Study the drawing (mm; zero at the part's minimum x, y, z) and answer. A direction names the side the tool comes from. Coordinates: 2 decimals unless noted, no trailing zeros. Order: outer loops, then holes, each group sorted by start corner. A loop starts at its lowest first (then second) coordinate and runs counter-clockwise, first axis right, second up. Notation, with made-up numbers: (53.5, 38) -> (59.5, 38) arc R27 cw to (59.5, 69) -> close; hole circle Ø11 at (53.5, 31). An arc over 180 degrees is marked (long way). One line per question, with ' | ' between items.
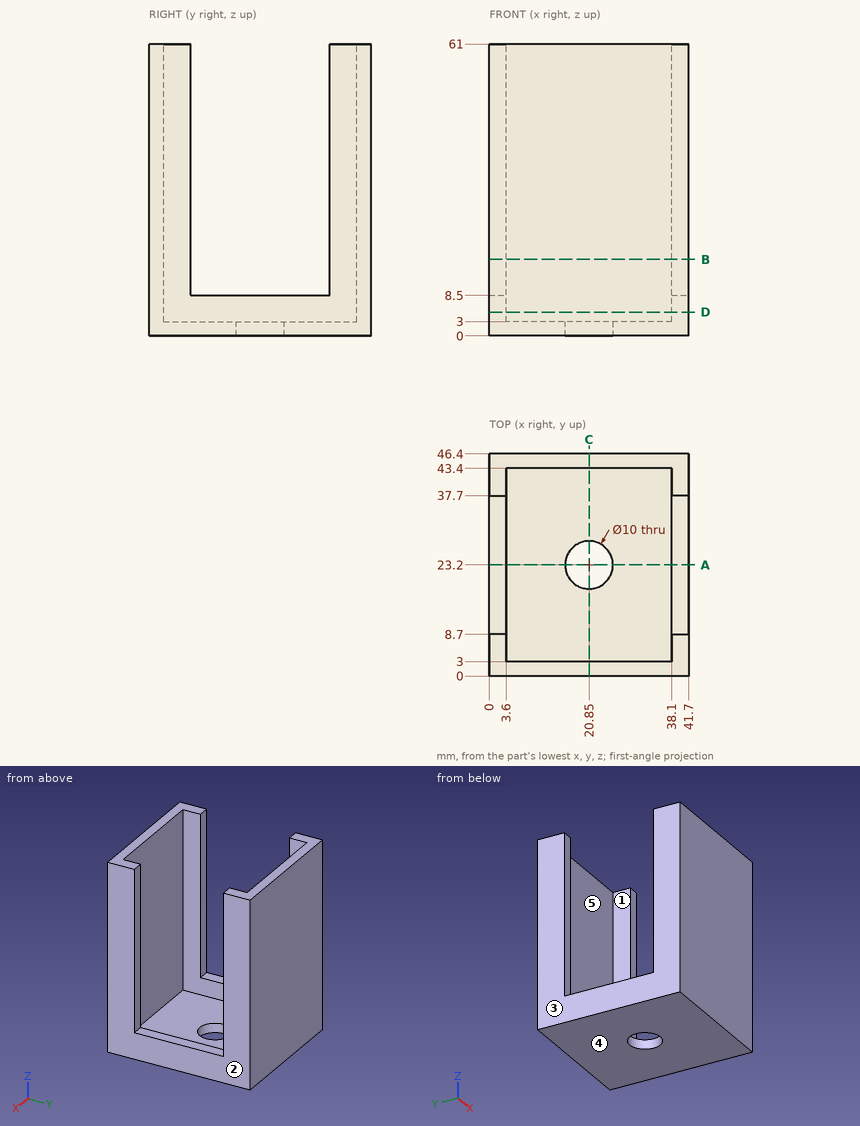
Item 1: Section A-A, the plane y = 23.2 is taken. Give the vertices of the cut face in (x, z), plus the area to 3 significant figures.
Computed values:
outline: (0, 0) -> (15.85, 0) -> (15.85, 3) -> (3.6, 3) -> (3.6, 8.5) -> (0, 8.5) -> close; (25.85, 0) -> (41.7, 0) -> (41.7, 8.5) -> (38.1, 8.5) -> (38.1, 3) -> (25.85, 3) -> close | area: 135 mm^2
Item 2: Section B-B, the plane z = 16 is taken. Give the vertices of the cut face in (x, y).
Computed values:
outline: (0, 0) -> (41.7, 0) -> (41.7, 8.7) -> (38.1, 8.7) -> (38.1, 3) -> (3.6, 3) -> (3.6, 8.7) -> (0, 8.7) -> close; (0, 37.7) -> (3.6, 37.7) -> (3.6, 43.4) -> (38.1, 43.4) -> (38.1, 37.7) -> (41.7, 37.7) -> (41.7, 46.4) -> (0, 46.4) -> close
Item 3: Each of these flat-tipped pins is pushed along its axis until it touches: pin 1 Ø3 at (x, y) = (2, 26.5) entering from +Z; pin 2 Ø8 at (x, y) = (27, 27) entering from +Z. Where does it stop, or does it pass through?
Computed values:
pin 1: stops at z = 8.5 | pin 2: stops at z = 3
Item 4: Section C-C, the plane x = 20.85 is taken. Give the vertices of the cut face in (y, z), plus the area to 3 significant figures.
Computed values:
outline: (0, 0) -> (18.2, 0) -> (18.2, 3) -> (3, 3) -> (3, 61) -> (0, 61) -> close; (28.2, 0) -> (46.4, 0) -> (46.4, 61) -> (43.4, 61) -> (43.4, 3) -> (28.2, 3) -> close | area: 457 mm^2
Item 5: Section D-D, the plane z = 5 is taken. Give the vertices of the cut face in (x, y), plus the area to 3 significant figures.
Computed values:
outline: (0, 0) -> (41.7, 0) -> (41.7, 46.4) -> (0, 46.4) -> close; hole (3.6, 3) -> (38.1, 3) -> (38.1, 43.4) -> (3.6, 43.4) -> close | area: 541 mm^2
Item 6: Find the intervals of material crossed by L1, parallel to Y at x = 8.5, z = 38.5; L2, parallel to Y at x = 20.85, z = 0.8; L3, parallel to X at y = 23, z = 1, in increasing order.
Computed values:
L1: y = 0 to 3, 43.4 to 46.4 | L2: y = 0 to 18.2, 28.2 to 46.4 | L3: x = 0 to 15.85, 25.85 to 41.7
Item 7: Determine the mould class of the marked faces 3, 4 and 5 for opening direction X: pulls with the +X half, pulls with the -X half, needs draft (parallel to the pull), parting line crosses it, or undercut.
Computed values:
face 3: pulls with the -X half | face 4: needs draft | face 5: undercut
Item 8: For the marked faces 1 and 2, determine the directions among +Z, -Z, +X, -X, +Y, -Y from which every point of the face is accessible in a straight line to the end or side of a thin tool.
Computed values:
face 1: +Z | face 2: +Z, -Z, +X, +Y, -Y
